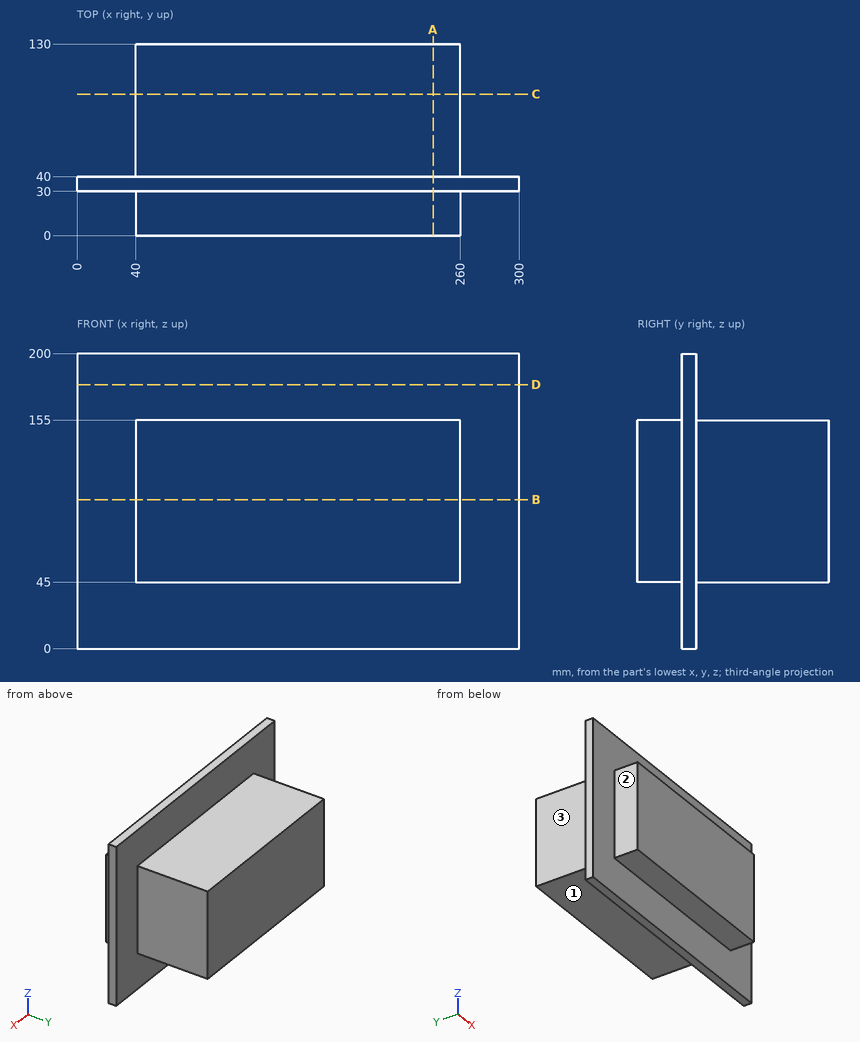
Print and shaded views of the part. All mm, measured from the part's lowest x, y and z. A direction names the side the tool comes from. Coordinates: 2 decimals unless noted, no trailing zeros. Order: outer loops, then holes, each group sorted by start corner. A loop starts at its lowest first (then second) coordinate and runs counter-clockwise, first axis right, second up. Notation, with made-up numbers: (25.5, -15) -> (76.5, -15) arc R29 cw to (76.5, 9) -> close; hole circle Ø11 at (32, -3). An arc over 180 degrees is marked (long way). Answer as a JSON object with one key per item and string values. Group by question number.
1) Cut at C-C, the plane y = 96. Write the cut outline in (x, z), then the cut area to 3 significant figures.
2) Cut at A-A, the plane x = 241.5. Write the cut outline in (y, z).
3) Flat gauge pins, fed straight in: pin 1 (10 mm diameter, centred on x = 152.5, y = 97.5, fed in from +Z); pin 2 (5 mm diameter, centred on x = 123, z = 159.5, fed in from -Y); pin 3 (12 mm diameter, centred on y = 51.5, z = 55.5, fed in from +X). Where does each tip first touch, or does it go through?
4) Cut at B-B, the plane z = 101. Write the cut outline in (x, y), then the cut area to 3 significant figures.
5) Drill centre lines: L1, parallel to Y at x = 201, z = 22.5; L2, parallel to Z at x = 212, y = 117.5; L3, parallel to X at y = 81, z = 125. Where is each one in solid material? Low to high.
6) Which spindle directions (+Z, -Z, +X, -X, +Y, -Y) get a long thin tool onto all of the face, cutting with end or side? Do the marked faces 1, 2 and 3. Say none if no direction does.
7) Cut at D-D, the plane z = 179. Write the cut outline in (x, y), then the cut area to 3 significant figures.
Check values:
{
 "1": {"outline": "(40, 45) -> (260, 45) -> (260, 155) -> (40, 155) -> close", "area": "24,200 mm²"},
 "2": {"outline": "(0, 45) -> (30, 45) -> (30, 0) -> (40, 0) -> (40, 45) -> (130, 45) -> (130, 155) -> (40, 155) -> (40, 200) -> (30, 200) -> (30, 155) -> (0, 155) -> close"},
 "3": {"pin 1": "stops at z = 155", "pin 2": "stops at y = 30", "pin 3": "stops at x = 260"},
 "4": {"outline": "(0, 30) -> (40, 30) -> (40, 0) -> (260, 0) -> (260, 30) -> (300, 30) -> (300, 40) -> (260, 40) -> (260, 130) -> (40, 130) -> (40, 40) -> (0, 40) -> close", "area": "29,400 mm²"},
 "5": {"L1": "y = 30 to 40", "L2": "z = 45 to 155", "L3": "x = 40 to 260"},
 "6": {"face 1": "-Z, +X, -X, +Y", "face 2": "+Z, -Z, -X, -Y", "face 3": "+Z, -Z, -X, +Y"},
 "7": {"outline": "(0, 30) -> (300, 30) -> (300, 40) -> (0, 40) -> close", "area": "3,000 mm²"}
}
